from build123d import *

# Parameters (mm, degrees)
TAGLIO_ESTRUSIONE1_DEPTH      = 21.0000001
TAGLIO_ESTRUSIONE1_DEPTH_BACK = 21.0000001
TAGLIO_ESTRUSIONE2_DEPTH      = 21.0000001
TAGLIO_ESTRUSIONE2_DEPTH_BACK = 21.0000001


with BuildPart() as part:
    # Schizzo1 → Rivoluzione1 (revolve)
    with BuildSketch(Plane.XY, mode=Mode.PRIVATE) as rivoluzione1_sk:
        with BuildLine():
            Line((20, 26.666666667), (20, 0))
            Line((20, 0), (17.5, 0))
            Line((17.5, 0), (17.5, 27.862996478))
            ThreePointArc((17.5, 27.862996478), (17.044466296, 29.948140619), (15.760869565, 31.653343386))
            ThreePointArc((15.760869565, 31.653343386), (8.40518297, 35.991238731), (0, 37.5))
            Line((0, 37.5), (0, 40))
            ThreePointArc((0, 40), (8.432740427, 38.631554615), (16, 34.666666667))
            ThreePointArc((16, 34.666666667), (18.94427191, 31.138802622), (20, 26.666666667))
        make_face()
    revolve(rivoluzione1_sk.sketch.rotate(Axis((0, 0, 0), (0, 1, 0)), 90), axis=Axis((0, 0, 0), (0, 1, 0)))  # turned: the seam where the file's is

    # Schizzo2 → Taglio-Estrusione1 (cut, two sides)
    with BuildSketch(Plane.XY) as taglio_estrusione1_sk:
        with BuildLine():
            Line((2.5, 22.5), (2.5, 7.5))
            ThreePointArc((2.5, 7.5), (0, 5), (-2.5, 7.5))
            Line((-2.5, 7.5), (-2.5, 22.5))
            ThreePointArc((-2.5, 22.5), (0, 25), (2.5, 22.5))
        make_face()
    extrude(amount=TAGLIO_ESTRUSIONE1_DEPTH, mode=Mode.SUBTRACT)
    extrude(taglio_estrusione1_sk.sketch, amount=-TAGLIO_ESTRUSIONE1_DEPTH_BACK, mode=Mode.SUBTRACT)

    # Schizzo3 → Taglio-Estrusione2 (cut, two sides)
    with BuildSketch(Plane(origin=(0, 0, 0), x_dir=(0, 0, -1), z_dir=(1, 0, 0))) as taglio_estrusione2_sk:
        with BuildLine():
            Line((2.5, 20), (2.5, 5))
            ThreePointArc((2.5, 5), (0, 2.5), (-2.5, 5))
            Line((-2.5, 5), (-2.5, 20))
            ThreePointArc((-2.5, 20), (0, 22.5), (2.5, 20))
        make_face()
    extrude(amount=TAGLIO_ESTRUSIONE2_DEPTH, mode=Mode.SUBTRACT)
    extrude(taglio_estrusione2_sk.sketch, amount=-TAGLIO_ESTRUSIONE2_DEPTH_BACK, mode=Mode.SUBTRACT)


solid = part.part
Could you check a few things on this model? Use its own coordinates, in mm. A direction names the side the tool comes from. Round coordinates to 2 decimals unless told otherwise and drop trailing zeros. Order: outer loops, then holes, each group sorted by start corner. A loop starts at its lowest first (then second) coordinate and runs counter-clockwise, first axis right, second up.
(1) Which directions (+Z, -Z, +X, -X, +Y, -Y) give clear straight access to the entire face, cutting with the end or side of a thin tool? Please do faces 1 (the cylindrical face through (15.526, 14.127, -8.075)), 2 (the flat face through (2.5, 15, -19)), 3 (the cylindrical face through (-6.007, 13.147, -19.076)), 4 (the flat face through (19, 12, 2.5)).
Response values:
face 1: -Y
face 2: +Z, -Z
face 3: +Y, -Y
face 4: +X, -X
(2) Imagine slicing it at A-A (x = 0). Write out the boundary of the cut face in (y, z).
Response values:
outline: (0, -20) - (5, -20) - (5, -17.5) - (0, -17.5) - close; (0, 17.5) - (5, 17.5) - (5, 20) - (0, 20) - close; (25, -20) - (26.67, -20) arc R10 ccw to (34.67, -16) arc R26.67 ccw to (34.67, 16) arc R10 ccw to (26.67, 20) - (25, 20) - (25, 17.5) - (27.86, 17.5) arc R5 cw to (31.65, 15.76) arc R24.17 cw to (31.65, -15.76) arc R5 cw to (27.86, -17.5) - (25, -17.5) - close
(3) Imagine slicing it at B-B (y = 18). Write out the boundary of the cut face in (x, z), plus the area to 3 significant figures.
Response values:
outline: (-19.84, -2.5) arc R20 ccw to (-2.5, -19.84) - (-2.5, -17.32) arc R17.5 cw to (-17.32, -2.5) - close; (-19.84, 2.5) - (-17.32, 2.5) arc R17.5 cw to (-2.5, 17.32) - (-2.5, 19.84) arc R20 ccw to start; (2.5, -19.84) arc R20 ccw to (19.84, -2.5) - (17.32, -2.5) arc R17.5 cw to (2.5, -17.32) - close; (2.5, 17.32) arc R17.5 cw to (17.32, 2.5) - (19.84, 2.5) arc R20 ccw to (2.5, 19.84) - close
area: 244 mm2
(4) Please list where these lines run through material, in increasing order: line 1 along Z through (x, y) = (-0.5, 5); line 2 along Z through (x, y) = (-10, 6); line 3 along X through (y, z) = (7.5, 17.5).
Response values:
line 1: z = -19.99 to -17.49, 17.49 to 19.99
line 2: z = -17.32 to -14.36, 14.36 to 17.32
line 3: x = -9.68 to -2.5, 2.5 to 9.68
(5) Imagine slicing it at C-C (z = 0). Write out the boundary of the cut face in (x, y), plus the area to 3 significant figures.
Response values:
outline: (-20, 0) - (-17.5, 0) - (-17.5, 2.5) - (-20, 2.5) - close; (-20, 22.5) - (-17.5, 22.5) - (-17.5, 27.86) arc R5 cw to (-15.76, 31.65) arc R24.17 cw to (15.76, 31.65) arc R5 cw to (17.5, 27.86) - (17.5, 22.5) - (20, 22.5) - (20, 26.67) arc R10 ccw to (16, 34.67) arc R26.67 ccw to (-16, 34.67) arc R10 ccw to (-20, 26.67) - close; (17.5, 0) - (20, 0) - (20, 2.5) - (17.5, 2.5) - close
area: 154 mm2
(6) I'm going to push flat-ended pins straight in: pin 1 (1.3 mm diameter, centred on x = -19, y = 13, fed in from +Z); pin 2 (1 mm diameter, centred on x = -7, z = -10, fed in from +Y); pin 3 (0.8 mm diameter, centred on x = 18, y = 9.5, fed in from -Z). Where does each tip first touch, or does it pass through?
Response values:
pin 1: stops at z = 7.95
pin 2: stops at y = 37.29
pin 3: stops at z = -9.5
(7) If we mould it in two halves opening along Y, with no side actions, what happens to faces 5 (the flat face through (18, 0, 0)), 6 (the cylindrical face through (0, 25, 19)), 7 (the flat face through (-2.5, 15, -19))? For each: released by +Y, released by -Y, zero draft, split by the parting line, or undercut.
Response values:
face 5: released by -Y
face 6: undercut
face 7: undercut
(8) Imagine slicing it at D-D (y = 6). Write out the boundary of the cut face in (x, z), plus the area to 3 significant figures.
Response values:
outline: (-19.84, -2.5) arc R20 ccw to (-2, -19.9) - (-2, -17.39) arc R17.5 cw to (-17.32, -2.5) - close; (-19.84, 2.5) - (-17.32, 2.5) arc R17.5 cw to (-2, 17.39) - (-2, 19.9) arc R20 ccw to start; (2, -19.9) arc R20 ccw to (19.84, -2.5) - (17.32, -2.5) arc R17.5 cw to (2, -17.39) - close; (2, 17.39) arc R17.5 cw to (17.32, 2.5) - (19.84, 2.5) arc R20 ccw to (2, 19.9) - close
area: 249 mm2
